Print and shaded views of the part. All mm, measured from the part's lowest x, y and z. A direction names the side the tool comes from. Round coordinates to 2 decimals unless told otherwise and drop trailing zeros. Write each loop counter-clockwise with the first axis right and the second up, starting at its lowest first coordinate (ties: lowest second). Pieces come first, ordered by that corner, then holes. Notation, with made-up numbers: M 40,44.25 L 99,44.25 A16 ccw 99,53.25 Z; hole C 46,79.25 d5. An arc over 180 degrees is marked long. Write item = value, one per line. Start each with the question number.
Q1. Band-saw the part on B-B on y = 24. Write the cut outline in (x, z).
Q2. Band-saw the part on D-D on x = 28. Write the cut outline in (y, z), plus the area to 3 significant figures.
Q3. Pull direction Z, two halves, no side cores. Call the marked faces 4, 5 and 6: released by +Z, released by -Z, zero draft, split by the parting line, or undercut.
Q4. Probe L1, parallel to X at y = 5.5, z = 20.5; L2, parallel to Z at x = 60, y = 8.5; L3, parallel to X at y = 8.5, z = 25. List the from-to ranges inside material, lowest first.
Q5. Band-saw the part on C-C on y = 7. State how many separate pieces and enclosed holes the cut face has.
Q6. Tool access for the marked faces 1, 2 and 3: list every direction of +Z, -Z, +X, -X, +Y, -Y with a clear straight run to the whole face (end or side of a thin tool).
Q7. Drop flat-ended pins along their axis: P1, Ø1.5, axis at y = 2, z = 10, coming from the -X side; P2, Ø1.5, axis at x = 66.5, z = 55.5, coming from the -Y side; P3, Ø3, axis at x = 5.904, z = 61.5, coming from the +Y side; P4, Ø1.1, axis at x = 73.5, y = 27.5, coming from the -Z side. Give the stop position or say it passes through.
Q8. Band-saw the part on A-A on z = 13. Write the cut outline in (x, y), plus the area to 3 significant figures.
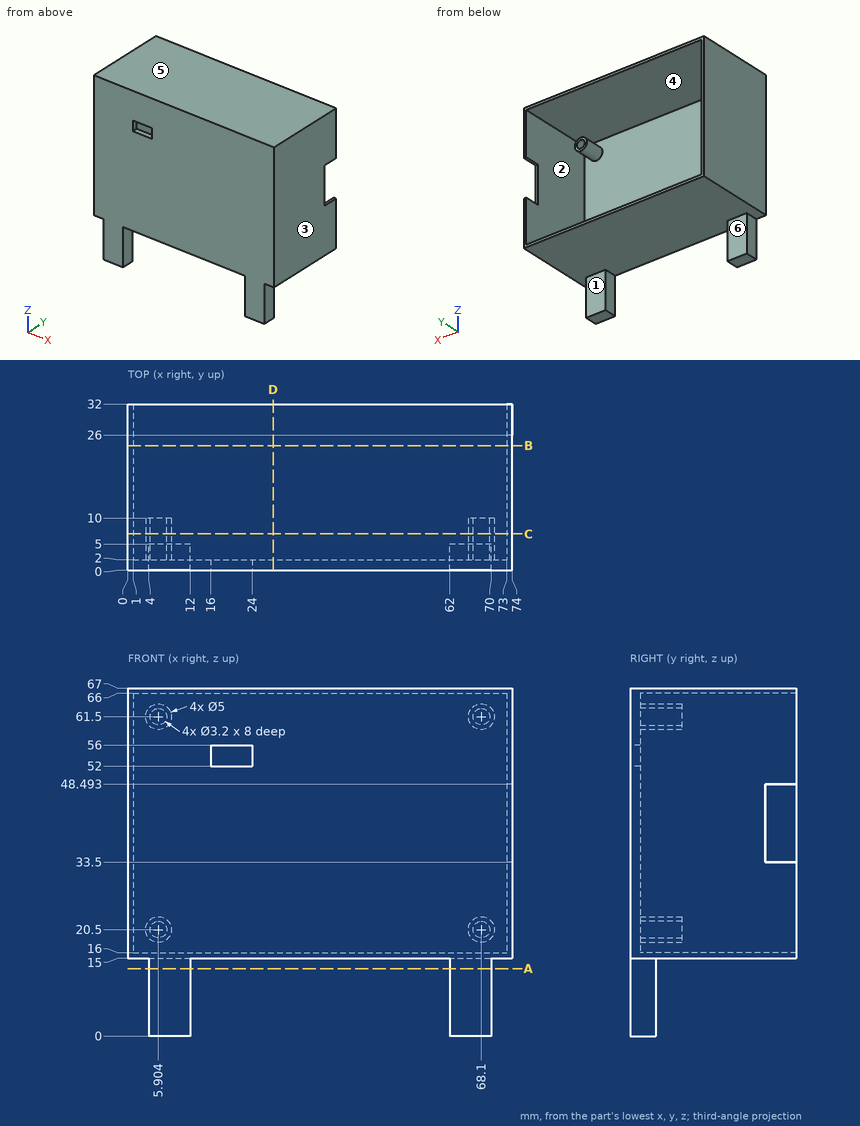
Conclusion:
q1.outline = M 0,15 L 74,15 L 74,67 L 0,67 Z; hole M 1,16 L 73,16 L 73,66 L 1,66 Z
q2.outline = M 0,15 L 32,15 L 32,16 L 2,16 L 2,66 L 32,66 L 32,67 L 0,67 Z
q2.area = 164 mm^2
q3.face_4 = undercut
q3.face_5 = released by +Z
q3.face_6 = zero draft
q4.L1 = 0 to 1, 3.4 to 4.3, 7.5 to 8.4, 65.6 to 66.5, 69.7 to 70.6, 73 to 74
q4.L2 = 15 to 16, 66 to 67
q4.L3 = 0 to 1, 73 to 74
q5.separate_pieces = 5
q5.enclosed_holes = 5
q6.face_1 = -Z, +X, -X, +Y
q6.face_2 = +Y
q6.face_3 = +Z, -Z, +X, +Y, -Y
q7.P1 = 4
q7.P2 = 0
q7.P3 = 2
q7.P4 = 15
q8.outline = M 4,0 L 12,0 L 12,5 L 4,5 Z; M 62,0 L 70,0 L 70,5 L 62,5 Z
q8.area = 80.0 mm^2
